from build123d import *

# Parameters (mm, degrees)
SKETCH1_R           = 2
BOSS_EXTRUDE1_DEPTH = 5
SKETCH2_W           = 7.9
SKETCH2_H           = 15
CUT_EXTRUDE1_DEPTH  = 10
CUT_EXTRUDE2_DEPTH  = 10


with BuildPart() as part:
    # Sketch1 → Boss-Extrude1 (new body)
    with BuildSketch(Plane.XY):
        with BuildLine():
            ThreePointArc((5, 51), (0, 56), (-5, 51))
            Line((-5, 51), (-5, 44.72135955))
            ThreePointArc((-5, 44.72135955), (-31.819805153, 31.819805153), (-44.72135955, 5))
            Line((-44.72135955, 5), (-51, 5))
            ThreePointArc((-51, 5), (-56, 0), (-51, -5))
            Line((-51, -5), (-44.72135955, -5))
            ThreePointArc((-44.72135955, -5), (-31.819805153, -31.819805153), (-5, -44.72135955))
            Line((-5, -44.72135955), (-5, -51))
            ThreePointArc((-5, -51), (0, -56), (5, -51))
            Line((5, -51), (5, -44.72135955))
            ThreePointArc((5, -44.72135955), (31.819805153, -31.819805153), (44.72135955, -5))
            Line((44.72135955, -5), (51, -5))
            ThreePointArc((51, -5), (56, 0), (51, 5))
            Line((51, 5), (44.72135955, 5))
            ThreePointArc((44.72135955, 5), (31.819805153, 31.819805153), (5, 44.72135955))
            Line((5, 44.72135955), (5, 51))
        make_face()
        with Locations((0, 51)):
            Circle(SKETCH1_R, mode=Mode.SUBTRACT)
        with Locations((0, 42.5)):
            Circle(SKETCH1_R, mode=Mode.SUBTRACT)
        with Locations((0, -42.5)):
            Circle(SKETCH1_R, mode=Mode.SUBTRACT)
        with Locations((-42.5, 0)):
            Circle(SKETCH1_R, mode=Mode.SUBTRACT)
        with Locations((42.5, 0)):
            Circle(SKETCH1_R, mode=Mode.SUBTRACT)
        with Locations((-51, 0)):
            Circle(SKETCH1_R, mode=Mode.SUBTRACT)
        with Locations((51, 0)):
            Circle(SKETCH1_R, mode=Mode.SUBTRACT)
        with Locations((0, -51)):
            Circle(SKETCH1_R, mode=Mode.SUBTRACT)
    extrude(amount=BOSS_EXTRUDE1_DEPTH)

    # Sketch2 → Cut-Extrude1 (cut)
    with BuildSketch(Plane(origin=(0, 0, 0), x_dir=(-1, 0, 0), z_dir=(0, 0, -1))):
        with Locations((0, -17.6)):
            Rectangle(SKETCH2_W, SKETCH2_H)
    extrude(amount=-CUT_EXTRUDE1_DEPTH, mode=Mode.SUBTRACT)

    # Sketch3 → Cut-Extrude2 (cut)
    with BuildSketch(Plane(origin=(0, 0, 0), x_dir=(-1, 0, 0), z_dir=(0, 0, -1))):
        with BuildLine():
            Line((-19, 18), (-19, -8))
            ThreePointArc((-19, -8), (-23, -12), (-27, -8))
            Line((-27, -8), (-27, 18))
            ThreePointArc((-27, 18), (-23, 22), (-19, 18))
        make_face()
    extrude(amount=-CUT_EXTRUDE2_DEPTH, mode=Mode.SUBTRACT)


solid = part.part
Source: CAD feature listing. Evaluate the final solid. Frame: model axes, mm. A direction names the side the tool comes from. Coordinates: 2 decimals unless noted, no trailing zeros. Write each loop counter-clockwise with the first axis right and the second up, starting at its lowest first coordinate (ties: lowest second). Pieces come first, ordered by that corner, then holes. Notation, with made-up numbers: M -18.5,-36.75 L 17.5,-36.75 A13 cw 17.5,-28.75 Z; hole C 27.25,49 d1. An arc over 180 degrees is marked long. Use a Markdown table: item, result.
1) Mould query, pull axis Y, two halves, no side actions, for faces 6 (the flat face through (27, 5, 2)), 7 (the cylindrical face through (-32.119, -31.518, 2.465)), 8 (the cylindrical face through (32.119, 31.518, 2.465)). Classes: pulls with the +Y half, pulls with the -Y half, needs draft (parallel to the pull), parting line crosses it, or undercut.
Conclusion:
| item | result |
|---|---|
| face 6 | undercut |
| face 7 | pulls with the -Y half |
| face 8 | pulls with the +Y half |
2) Section C-C, the plane x = 22. Output: boundary loops of the cut face in (y, z).
Conclusion:
| item | result |
|---|---|
| outline | M -39.26,0 L -11.87,0 L -11.87,5 L -39.26,5 Z; M 21.87,0 L 39.26,0 L 39.26,5 L 21.87,5 Z |
3) First-contact query: pin 1 Ø1.5 at (x, z) = (-47.5, 2) entering from -Y; pin 2 Ø1.5 at (x, z) = (2, 3.5) entering from +Y; pin 3 Ø2.5 at (y, z) = (47, 2) entering from +X. Flat tips, straight axial feed; report the tip coordinate or a pass-through.
Conclusion:
| item | result |
|---|---|
| pin 1 | stops at y = -5 |
| pin 2 | stops at y = 55.84 |
| pin 3 | stops at x = 5 |
4) Reachability of faces 1 (the flat face through (-5, -48, 2)), 2 (the flat face through (5, -48, 2)), 3 (the flat face through (3.95, -18, 2)), 4 (the flat face through (5, 48, 2)), 5 (the flat face through (-1, 1, 0)) from +Z, -Z, +X, -X, +Y, -Y: full face, straight path, thin tool, end or side. Return the list, or none.
Conclusion:
| item | result |
|---|---|
| face 1 | +Z, -Z, -X, -Y |
| face 2 | +Z, -Z, +X, -Y |
| face 3 | +Z, -Z |
| face 4 | +Z, -Z, +X, +Y |
| face 5 | -Z, +X, -X, +Y, -Y |
5) Section B-B, the plane z = 1.5. Give the number of separate pieces and of enclosed holes in the cut face, then the cut area to 3 significant figures.
Conclusion:
| item | result |
|---|---|
| separate pieces | 1 |
| enclosed holes | 10 |
| area | 6,290 mm^2 |
6) Ray query, L1, parallel to Y at x = 0, z = 1.4; L2, parallel to X at y = -0.5, z = 3.7; L3, parallel to Y at x = -51, z = 2.2. Return the intervals inside material, ascending.
Conclusion:
| item | result |
|---|---|
| L1 | y = -56 to -53, -49 to -44.5, -40.5 to -25.1, -10.1 to 40.5, 44.5 to 49, 53 to 56 |
| L2 | x = -55.97 to -52.94, -49.06 to -44.44, -40.56 to 19, 27 to 40.56, 44.44 to 49.06, 52.94 to 55.97 |
| L3 | y = -5 to -2, 2 to 5 |
7) Section D-D, the plane y = -19. Output: boundary loops of the cut face in (x, z).
Conclusion:
| item | result |
|---|---|
| outline | M -40.79,0 L -3.95,0 L -3.95,5 L -40.79,5 Z; M 3.95,0 L 40.79,0 L 40.79,5 L 3.95,5 Z |
8) Section A-A, the plane x = 0. Output: boundary loops of the cut face in (y, z).
Conclusion:
| item | result |
|---|---|
| outline | M -56,0 L -53,0 L -53,5 L -56,5 Z; M -49,0 L -44.5,0 L -44.5,5 L -49,5 Z; M -40.5,0 L -25.1,0 L -25.1,5 L -40.5,5 Z; M -10.1,0 L 40.5,0 L 40.5,5 L -10.1,5 Z; M 44.5,0 L 49,0 L 49,5 L 44.5,5 Z; M 53,0 L 56,0 L 56,5 L 53,5 Z |
